from build123d import *

# Parameters (mm, degrees)
EXTRUSION1_DEPTH      = 15
ESQUISSE2_R           = 48
EXTRUSION2_DEPTH      = 4
EXTRUSION2_DEPTH_BACK = 19
CONG_1_R              = 2
EXTRUSION5_DEPTH      = 25
ESQUISSE6_W           = 12
ESQUISSE6_H           = 14
ESQUISSE6_W_2         = 10
ESQUISSE6_H_2         = 12
EXTRUSION6_DEPTH      = 10


with BuildPart() as part:
    # Esquisse1 → Extrusion1 (new body)
    with BuildSketch(Plane(origin=(0, 0, 0), x_dir=(1, 0, 0), z_dir=(0, 1, 0))):
        Polygon((-7.5, 100), (7.5, 100), (7.5, 50), (39.104688576, 18.395311424), (32.033620764, 11.324243612), (15, 28.357864376), (15, 0), (-15, 0), (-15, 28.357864376), (-32.033620764, 11.324243612), (-39.104688576, 18.395311424), (-7.5, 50), align=None)
    extrude(amount=EXTRUSION1_DEPTH)

    # Esquisse2 → Extrusion2 (add, two sides)
    with BuildSketch(Plane(origin=(0, 15, 0), x_dir=(1, 0, 0), z_dir=(0, 1, 0))) as extrusion2_sk:
        with Locations((0, 50)):
            Circle(ESQUISSE2_R)
    extrude(amount=EXTRUSION2_DEPTH)
    extrude(extrusion2_sk.sketch, amount=-EXTRUSION2_DEPTH_BACK)

    # Congé1
    cong_1_edges = [part.edges().sort_by_distance(p)[0] for p in [
        (-48, -4, -50),
        (-48, 19, -50),
    ]]
    fillet(cong_1_edges, radius=CONG_1_R)

    # Esquisse5 → Extrusion5 (add)
    with BuildSketch(Plane(origin=(-10.354688576, 0, 10.354688576), x_dir=(0.707106781, 0, 0.707106781), z_dir=(-0.707106781, 0, 0.707106781))):
        with BuildLine():
            Line((-39.658639918, 3.5), (-39.658639918, 10))
            ThreePointArc((-39.658639918, 10), (-38.926406871, 11.767766953), (-37.158639918, 12.5))
            Line((-37.158639918, 12.5), (-34.158639918, 12.5))
            ThreePointArc((-34.158639918, 12.5), (-32.390872965, 11.767766953), (-31.658639918, 10))
            Line((-31.658639918, 10), (-31.658639918, 3.5))
            Line((-31.658639918, 3.5), (-39.658639918, 3.5))
        make_face()
        with BuildLine():
            Line((-37.658639918, 10), (-37.658639918, 5.5))
            Line((-37.658639918, 5.5), (-33.658639918, 5.5))
            Line((-33.658639918, 5.5), (-33.658639918, 10))
            ThreePointArc((-33.658639918, 10), (-33.805086528, 10.353553391), (-34.158639918, 10.5))
            Line((-34.158639918, 10.5), (-37.158639918, 10.5))
            ThreePointArc((-37.158639918, 10.5), (-37.512193309, 10.353553391), (-37.658639918, 10))
        make_face(mode=Mode.SUBTRACT)
    extrude(amount=EXTRUSION5_DEPTH)

    # Esquisse6 → Extrusion6 (add)
    with BuildSketch(Plane(origin=(0, 0, -100), x_dir=(-1, 0, 0), z_dir=(0, 0, -1))):
        with Locations((0, 7.5)):
            Rectangle(ESQUISSE6_W, ESQUISSE6_H)
        with Locations((0, 7.5)):
            Rectangle(ESQUISSE6_W_2, ESQUISSE6_H_2, mode=Mode.SUBTRACT)
    extrude(amount=EXTRUSION6_DEPTH)


solid = part.part
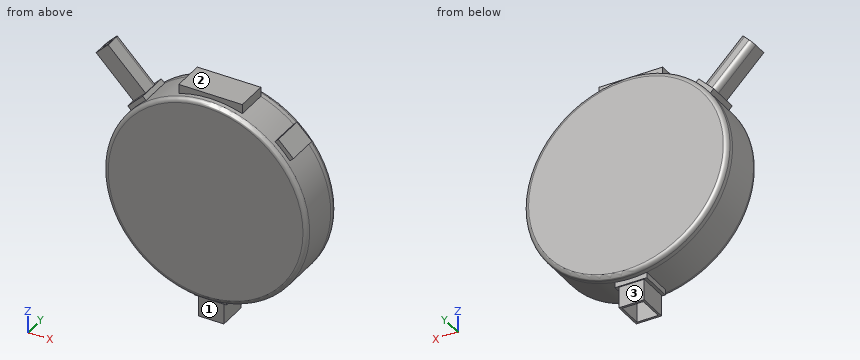
Can you work these out from the model? Positions are in its coordinate system, mm. Face numbers are marked on the shaded views. A direction names the side the tool comes from. Coordinates: 2 decimals unless noted, no trailing zeros. Order: outer loops, then holes, each group sorted by start corner. A loop starts at its lowest first (then second) coordinate and runs counter-clockwise, first axis right, second up. Notation, with made-up numbers: (70, -35) - (82, -35) arc R13 ccw to (82, -16) - close; hole circle Ø8 at (28.25, 3.5). An arc over 180 degrees is marked (long way). Answer as a JSON object with one key per item and string values. Group by question number.
Q1. On a 3-axis mill with a long thin cutter (end or side, diameter ignored), from which of +Z, -Z, +X, -X, +Y, -Y can I reach the whole of each face in a straight line? I mean the marked faces 1, 2 and 3. Say none if no direction works.
Q2. Imagine slicing it at B-B (z = -50). Please give me the cut outline in (x, y).
Q3. I need wall thicknesses on line 1 (Y direction, x = -40, z = -8.5); line 2 (X direction, y = 6.25, z = -103.5); line 3 (Y direction, x = -45, z = -39). Which ranges of each line are inside material? Lowest first, please. Write a range as from..to.
Q4. Imagine slicing it at A-A (x = 0). Please give me the cut outline in (y, z), and give its area (3 significant figures).
Q5. Will these pins go through, and if not, where does the flat tip stop? P1, Ø8, axis at y = 5, z = -106.5, coming from the -X side; P2, Ø6, axis at x = -42.5, z = -1, coming from the +Y side; P3, Ø4.5, axis at x = 33, z = -16.5, coming from the +Y side; P4, Ø1.3, axis at y = 7, z = -99.5, coming from the -X side.
Determined:
{
 "1": {"face 1": "-Z, +X, -X, -Y", "face 2": "+Z, +X, +Y, -Y", "face 3": "-Z, +X, -X, +Y"},
 "2": {"outline": "(-48, -2) arc R2 ccw to (-46, -4) - (46, -4) arc R2 ccw to (48, -2) - (48, 17) arc R2 ccw to (46, 19) - (-46, 19) arc R2 ccw to (-48, 17) - close"},
 "3": {"line 1": "y = 3.5..5.5, 10.5..12.5", "line 2": "x = -6..-5, 5..6", "line 3": "y = -3.97..18.97"},
 "4": {"outline": "(-4, -96) arc R2 ccw to (-2, -98) - (0, -98) - (0, -100) - (0.5, -100) - (0.5, -110) - (1.5, -110) - (1.5, -100) - (13.5, -100) - (13.5, -110) - (14.5, -110) - (14.5, -100) - (15, -100) - (15, -98) - (17, -98) arc R2 ccw to (19, -96) - (19, -4) arc R2 ccw to (17, -2) - (15, -2) - (15, 0) - (0, 0) - (0, -2) - (-2, -2) arc R2 ccw to (-4, -4) - close", "area": "2,280 mm2"},
 "5": {"P1": "stops at x = -6", "P2": "stops at y = 12.47", "P3": "stops at y = 19", "P4": "stops at x = -7.5"}
}
